For this review, use the dimensioned drawing (mm, ordinates from the lowest corner) and the shaded views. A direction names the side the tool comes from. Give positions to 0.01 mm unless a question says otherwise; leave off trailing zeros. Write each loop counter-clockwise with the first axis right and the second up, starting at its lowest first coordinate (ties: lowest second). Pieces come first, ordered by that corner, then holes.
1) For P1, Ø4, axis at x = 25.5, z = 31.5, coming from the -Y side; P2, Ø6, axis at y = 32.5, z = 65.5, coming from the +X side; P3, Ø2, axis at x = 39.5, z = 34, coming from the +Y side (1 decimal); P4, Ø21, axis at x = 47.5, z = 85, coming from the +Y side, all flat-tipped, find the tip position at first contact; note any pin that passes through.
2) We need section D-D on z = 114.5. Give the boundary of the cut face in (x, y).
3) We need section C-C on y = 7. Give the boundary of the cut face in (x, z), and give its area (3 significant figures).
4) Draft analysis for pull direction Y (two halves, no side actions). For the marked faces 1, 2, 3 and 4, state which applies: pulls with the +Y half, pulls with the -Y half, needs draft (parallel to the pull), parting line crosses it, or undercut.
5) Machinability: for the marked faces 5, 6 and 7, which of the approach directions +Z, -Z, +X, -X, +Y, -Y give a long, thin tool a straight path to every point of the face, cutting with its end or side? Answer none if there is none.
6) Wall thickness on line 1 along Y through (x, z) = (26, 65); line 2 along Z through (x, y) = (70.5, 31); line 3 along Y through (x, z) = (62.5, 30): over which ranges is each line inside the solid? List them lowest first.
7) We need section A-A on z = 93.5. Give the boundary of the cut face in (x, y), and give its area (3 significant figures).
8) We need section B-B on x = 36.5. Give the boundary of the cut face in (y, z), and give its area (3 significant figures).
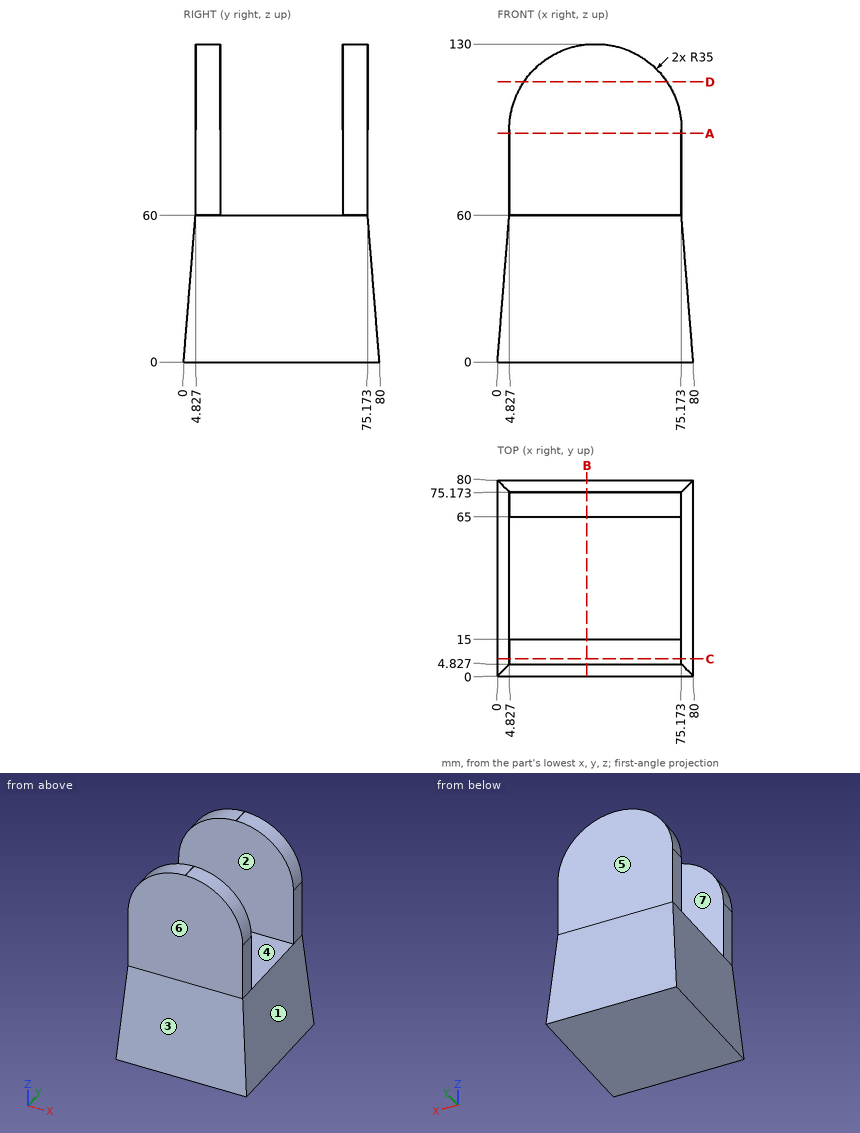
Results list:
1. P1: stops at y = 2.37
1. P2: passes through
1. P3: stops at y = 77.3
1. P4: stops at y = 75.17
2. outline: (10.76, 4.83) - (69.24, 4.83) - (69.24, 15) - (10.76, 15) - close; (10.76, 65) - (69.24, 65) - (69.24, 75.17) - (10.76, 75.17) - close
3. outline: (0, 0) - (80, 0) - (75.17, 60) - (75.17, 95) arc R35 ccw to (40.17, 130) - (39.83, 130) arc R35 ccw to (4.83, 95) - (4.83, 60) - close
3. area: 8,910 mm2
4. face 1: needs draft
4. face 2: undercut
4. face 3: pulls with the -Y half
4. face 4: undercut
5. face 5: +Z, +X, -X, +Y
5. face 6: +Z, +X, -X, -Y
5. face 7: +Z, +X, -X
6. line 1: y = 4.83 to 15, 65 to 75.17
6. line 2: z = 0 to 60
6. line 3: y = 2.41 to 77.59
7. outline: (4.83, 4.83) - (75.17, 4.83) - (75.17, 15) - (4.83, 15) - close; (4.83, 65) - (75.17, 65) - (75.17, 75.17) - (4.83, 75.17) - close
7. area: 1,430 mm2
8. outline: (0, 0) - (80, 0) - (75.17, 60) - (75.17, 129.84) - (65, 129.84) - (65, 60) - (15, 60) - (15, 129.84) - (4.83, 129.84) - (4.83, 60) - close
8. area: 5,930 mm2
